```python
from build123d import *

# Parameters (mm, degrees)
SKETCH1_W             = 20
SKETCH1_H             = 20
BOSS_EXTRUDE3_DEPTH   = 30
CUT_EXTRUDE11_REACH   = 39.417
SKETCH10_R            = 0.86
FILLET4_R             = 1
SKETCH12_W            = 2.7
SKETCH12_H            = 30
BOSS_EXTRUDE13_DEPTH  = 25
CUT_EXTRUDE13_REACH   = 51.237
SKETCH14_R            = 3.23
FILLET6_R             = 3
SKETCH16_W            = 2.7
SKETCH16_H            = 30
BOSS_EXTRUDE14_DEPTH  = 25
CUT_EXTRUDE14_REACH   = 51.237
SKETCH17_R            = 3.23
FILLET11_R            = 3
FILLET6_OF_MIRROR1_R  = 3
FILLET11_OF_MIRROR1_R = 3
FILLET12_R            = 1
CUT_EXTRUDE15_REACH   = 57
SKETCH18_R            = 1
CUT_EXTRUDE16_REACH   = 51.237
SKETCH20_R            = 1.98
SKETCH20_R_2          = 1.475
CUT_EXTRUDE17_REACH   = 56.668
SKETCH21_R            = 1.98
SKETCH21_R_2          = 1.475
SKETCH22_R            = 2.725
SKETCH22_R_2          = 3.23
CUT_EXTRUDE18_DEPTH   = 1.35
SKETCH23_R            = 2.725
SKETCH23_R_2          = 3.23
CUT_EXTRUDE19_DEPTH   = 1.35
CUT_EXTRUDE20_REACH   = 52.249
SKETCH24_W            = 8
SKETCH24_H            = 20
FILLET13_R            = 2


with BuildPart() as part:
    # Sketch1 → Boss-Extrude3 (new body)
    with BuildSketch(Plane(origin=(0, 0, 0), x_dir=(1, 0, 0), z_dir=(0, 1, 0))):
        Rectangle(SKETCH1_W, SKETCH1_H)
    extrude(amount=BOSS_EXTRUDE3_DEPTH)

    # Sketch10 → Cut-Extrude11 (cut, up to next)
    with BuildSketch(Plane(origin=(0, 0, -10), x_dir=(-1, 0, 0), z_dir=(0, 0, -1)), mode=Mode.PRIVATE) as cut_extrude11_sk1:
        with Locations((-5.88, 19.86)):
            Circle(SKETCH10_R)
    cut_extrude11_tool1 = extrude(cut_extrude11_sk1.sketch, amount=-CUT_EXTRUDE11_REACH, mode=Mode.PRIVATE) & part.part
    # Sketch10 → Cut-Extrude11 (cut, up to next)
    with BuildSketch(Plane(origin=(0, 0, -10), x_dir=(-1, 0, 0), z_dir=(0, 0, -1)), mode=Mode.PRIVATE) as cut_extrude11_sk2:
        with Locations((-5.92, 9.33)):
            Circle(SKETCH10_R)
    cut_extrude11_tool2 = extrude(cut_extrude11_sk2.sketch, amount=-CUT_EXTRUDE11_REACH, mode=Mode.PRIVATE) & part.part
    # Sketch10 → Cut-Extrude11 (cut, up to next)
    with BuildSketch(Plane(origin=(0, 0, -10), x_dir=(-1, 0, 0), z_dir=(0, 0, -1)), mode=Mode.PRIVATE) as cut_extrude11_sk3:
        Polygon((-1.75, 27.5), (1.75, 27.5), (1.75, 18), (7.3, 18), (7.3, 12), (1.75, 12), (1.75, 2.5), (-1.75, 2.5), (-1.75, 12), (-7.3, 12), (-7.3, 18), (-1.75, 18), align=None)
    cut_extrude11_tool3 = extrude(cut_extrude11_sk3.sketch, amount=-CUT_EXTRUDE11_REACH, mode=Mode.PRIVATE) & part.part
    add(cut_extrude11_tool1.solids().sort_by_distance((5.88, 19.86, -10))[0], mode=Mode.SUBTRACT)
    add(cut_extrude11_tool2.solids().sort_by_distance((5.92, 9.33, -10))[0], mode=Mode.SUBTRACT)
    add(cut_extrude11_tool3.solids().sort_by_distance((0, 15, -10))[0], mode=Mode.SUBTRACT)

    # Fillet4
    fillet4_edges = [part.edges().sort_by_distance(p)[0] for p in [
        (-1.75, 2.5, 0),
        (1.75, 2.5, 0),
        (1.75, 12, 0),
        (7.3, 12, 0),
        (7.3, 18, 0),
        (1.75, 18, 0),
        (1.75, 27.5, 0),
        (-1.75, 27.5, 0),
        (-1.75, 18, 0),
        (-7.3, 18, 0),
        (-7.3, 12, 0),
        (-1.75, 12, 0),
    ]]
    fillet(fillet4_edges, radius=FILLET4_R)

    # Sketch12 → Boss-Extrude13 (add)
    with BuildSketch(Plane.XY.offset(10)):
        with Locations((-8.65, 15)):
            Rectangle(SKETCH12_W, SKETCH12_H)
    boss_extrude13 = extrude(amount=BOSS_EXTRUDE13_DEPTH)

    # Sketch14 → Cut-Extrude13 (cut, up to next)
    with BuildSketch(Plane(origin=(-7.3, 0, 0), x_dir=(0, 0, -1), z_dir=(1, 0, 0)), mode=Mode.PRIVATE) as cut_extrude13_sk1:
        with Locations(Location((-29, 15, 0), (0, 0, 90))):
            Circle(SKETCH14_R)
    cut_extrude13_tool1 = extrude(cut_extrude13_sk1.sketch, amount=-CUT_EXTRUDE13_REACH, mode=Mode.PRIVATE) & part.part
    cut_extrude13 = cut_extrude13_tool1.solids().sort_by_distance((-7.3, 15, 29))[0]
    add(cut_extrude13, mode=Mode.SUBTRACT)

    # Fillet6
    fillet6_edges = [part.edges().sort_by_distance(p)[0] for p in [
        (-8.65, 0, 35),
        (-8.65, 30, 35),
    ]]
    fillet(fillet6_edges, radius=FILLET6_R)

    # Sketch16 → Boss-Extrude14 (add)
    with BuildSketch(Plane(origin=(0, 0, -10), x_dir=(-1, 0, 0), z_dir=(0, 0, -1))):
        with Locations((8.65, 15)):
            Rectangle(SKETCH16_W, SKETCH16_H)
    boss_extrude14 = extrude(amount=BOSS_EXTRUDE14_DEPTH)

    # Sketch17 → Cut-Extrude14 (cut, up to next)
    with BuildSketch(Plane(origin=(-7.3, 0, 0), x_dir=(0, 0, -1), z_dir=(1, 0, 0)), mode=Mode.PRIVATE) as cut_extrude14_sk1:
        with Locations((29, 15)):
            Circle(SKETCH17_R)
    cut_extrude14_tool1 = extrude(cut_extrude14_sk1.sketch, amount=-CUT_EXTRUDE14_REACH, mode=Mode.PRIVATE) & part.part
    cut_extrude14 = cut_extrude14_tool1.solids().sort_by_distance((-7.3, 15, -29))[0]
    add(cut_extrude14, mode=Mode.SUBTRACT)

    # Fillet11
    fillet11_edges = [part.edges().sort_by_distance(p)[0] for p in [
        (-8.65, 30, -35),
        (-8.65, 0, -35),
    ]]
    fillet(fillet11_edges, radius=FILLET11_R)

    # Mirror1: Boss-Extrude13, Cut-Extrude13, Boss-Extrude14, Cut-Extrude14 across plane
    add(boss_extrude13.mirror(Plane(origin=(0, 0, 0), x_dir=(0, 0, 1), z_dir=(1, 0, 0))))
    add(cut_extrude13.mirror(Plane(origin=(0, 0, 0), x_dir=(0, 0, 1), z_dir=(1, 0, 0))), mode=Mode.SUBTRACT)
    add(boss_extrude14.mirror(Plane(origin=(0, 0, 0), x_dir=(0, 0, 1), z_dir=(1, 0, 0))))
    add(cut_extrude14.mirror(Plane(origin=(0, 0, 0), x_dir=(0, 0, 1), z_dir=(1, 0, 0))), mode=Mode.SUBTRACT)

    # Fillet6 of Mirror1
    fillet6_of_mirror1_edges = [part.edges().sort_by_distance(p)[0] for p in [
        (8.65, 0, 35),
        (8.65, 30, 35),
    ]]
    fillet(fillet6_of_mirror1_edges, radius=FILLET6_OF_MIRROR1_R)

    # Fillet11 of Mirror1
    fillet11_of_mirror1_edges = [part.edges().sort_by_distance(p)[0] for p in [
        (8.65, 30, -35),
        (8.65, 0, -35),
    ]]
    fillet(fillet11_of_mirror1_edges, radius=FILLET11_OF_MIRROR1_R)

    # Fillet12
    fillet12_edges = [part.edges().sort_by_distance(p)[0] for p in [
        (0, 0, 10),
        (0, 30, 10),
        (0, 0, -10),
        (0, 30, -10),
    ]]
    fillet(fillet12_edges, radius=FILLET12_R)

    # Sketch18 → Cut-Extrude15 (cut, up to next)
    with BuildSketch(Plane(origin=(0, 0, -10), x_dir=(-1, 0, 0), z_dir=(0, 0, -1)), mode=Mode.PRIVATE) as cut_extrude15_sk1:
        with Locations((-3, 27)):
            Circle(SKETCH18_R)
    cut_extrude15_tool1 = extrude(cut_extrude15_sk1.sketch, amount=-CUT_EXTRUDE15_REACH, mode=Mode.PRIVATE) & part.part
    # Sketch18 → Cut-Extrude15 (cut, up to next)
    with BuildSketch(Plane(origin=(0, 0, -10), x_dir=(-1, 0, 0), z_dir=(0, 0, -1)), mode=Mode.PRIVATE) as cut_extrude15_sk2:
        with Locations((3, 3)):
            Circle(SKETCH18_R)
    cut_extrude15_tool2 = extrude(cut_extrude15_sk2.sketch, amount=-CUT_EXTRUDE15_REACH, mode=Mode.PRIVATE) & part.part
    cut_extrude15_1 = cut_extrude15_tool1.solids().sort_by_distance((3, 27, -10))[0]
    add(cut_extrude15_1, mode=Mode.SUBTRACT)
    cut_extrude15_2 = cut_extrude15_tool2.solids().sort_by_distance((-3, 3, -10))[0]
    add(cut_extrude15_2, mode=Mode.SUBTRACT)
    cut_extrude15 = cut_extrude15_1 + cut_extrude15_2  # Cut-Extrude15 as one shape, for the pattern or mirror that repeats it

    # Mirror2: Cut-Extrude15 across plane
    add(cut_extrude15.mirror(Plane(origin=(0, 0, 0), x_dir=(0, 0, 1), z_dir=(1, 0, 0))), mode=Mode.SUBTRACT)

    # Sketch20 → Cut-Extrude16 (cut, up to next)
    with BuildSketch(Plane.ZY.offset(-7.3), mode=Mode.PRIVATE) as cut_extrude16_sk1:
        with Locations((-13.25, 25.48)):
            Circle(SKETCH20_R)
    cut_extrude16_tool1 = extrude(cut_extrude16_sk1.sketch, amount=-CUT_EXTRUDE16_REACH, mode=Mode.PRIVATE) & part.part
    # Sketch20 → Cut-Extrude16 (cut, up to next)
    with BuildSketch(Plane.ZY.offset(-7.3), mode=Mode.PRIVATE) as cut_extrude16_sk2:
        with Locations((-13.25, 4.52)):
            Circle(SKETCH20_R)
    cut_extrude16_tool2 = extrude(cut_extrude16_sk2.sketch, amount=-CUT_EXTRUDE16_REACH, mode=Mode.PRIVATE) & part.part
    # Sketch20 → Cut-Extrude16 (cut, up to next)
    with BuildSketch(Plane.ZY.offset(-7.3), mode=Mode.PRIVATE) as cut_extrude16_sk3:
        with Locations((-29, 5.48)):
            Circle(SKETCH20_R_2)
    cut_extrude16_tool3 = extrude(cut_extrude16_sk3.sketch, amount=-CUT_EXTRUDE16_REACH, mode=Mode.PRIVATE) & part.part
    # Sketch20 → Cut-Extrude16 (cut, up to next)
    with BuildSketch(Plane.ZY.offset(-7.3), mode=Mode.PRIVATE) as cut_extrude16_sk4:
        with Locations((-29, 24.52)):
            Circle(SKETCH20_R_2)
    cut_extrude16_tool4 = extrude(cut_extrude16_sk4.sketch, amount=-CUT_EXTRUDE16_REACH, mode=Mode.PRIVATE) & part.part
    add(cut_extrude16_tool1.solids().sort_by_distance((7.3, 25.48, -13.25))[0], mode=Mode.SUBTRACT)
    add(cut_extrude16_tool2.solids().sort_by_distance((7.3, 4.52, -13.25))[0], mode=Mode.SUBTRACT)
    add(cut_extrude16_tool3.solids().sort_by_distance((7.3, 5.48, -29))[0], mode=Mode.SUBTRACT)
    add(cut_extrude16_tool4.solids().sort_by_distance((7.3, 24.52, -29))[0], mode=Mode.SUBTRACT)

    # Sketch21 → Cut-Extrude17 (cut, up to next)
    with BuildSketch(Plane(origin=(-7.3, 0, 7.3), x_dir=(0, 0, 1), z_dir=(-1, 0, 0)), mode=Mode.PRIVATE) as cut_extrude17_sk1:
        with Locations(Location((5.95, 25.48, 0), (0, 0, 180))):
            Circle(SKETCH21_R)
    cut_extrude17_tool1 = extrude(cut_extrude17_sk1.sketch, amount=CUT_EXTRUDE17_REACH, mode=Mode.PRIVATE) & part.part
    # Sketch21 → Cut-Extrude17 (cut, up to next)
    with BuildSketch(Plane(origin=(-7.3, 0, 7.3), x_dir=(0, 0, 1), z_dir=(-1, 0, 0)), mode=Mode.PRIVATE) as cut_extrude17_sk2:
        with Locations(Location((5.95, 4.52, 0), (0, 0, 180))):
            Circle(SKETCH21_R)
    cut_extrude17_tool2 = extrude(cut_extrude17_sk2.sketch, amount=CUT_EXTRUDE17_REACH, mode=Mode.PRIVATE) & part.part
    # Sketch21 → Cut-Extrude17 (cut, up to next)
    with BuildSketch(Plane(origin=(-7.3, 0, 7.3), x_dir=(0, 0, 1), z_dir=(-1, 0, 0)), mode=Mode.PRIVATE) as cut_extrude17_sk3:
        with Locations(Location((21.7, 5.48, 0), (0, 0, 180))):
            Circle(SKETCH21_R_2)
    cut_extrude17_tool3 = extrude(cut_extrude17_sk3.sketch, amount=CUT_EXTRUDE17_REACH, mode=Mode.PRIVATE) & part.part
    # Sketch21 → Cut-Extrude17 (cut, up to next)
    with BuildSketch(Plane(origin=(-7.3, 0, 7.3), x_dir=(0, 0, 1), z_dir=(-1, 0, 0)), mode=Mode.PRIVATE) as cut_extrude17_sk4:
        with Locations(Location((21.7, 24.52, 0), (0, 0, 180))):
            Circle(SKETCH21_R_2)
    cut_extrude17_tool4 = extrude(cut_extrude17_sk4.sketch, amount=CUT_EXTRUDE17_REACH, mode=Mode.PRIVATE) & part.part
    add(cut_extrude17_tool1.solids().sort_by_distance((-7.3, 25.48, 13.25))[0], mode=Mode.SUBTRACT)
    add(cut_extrude17_tool2.solids().sort_by_distance((-7.3, 4.52, 13.25))[0], mode=Mode.SUBTRACT)
    add(cut_extrude17_tool3.solids().sort_by_distance((-7.3, 5.48, 29))[0], mode=Mode.SUBTRACT)
    add(cut_extrude17_tool4.solids().sort_by_distance((-7.3, 24.52, 29))[0], mode=Mode.SUBTRACT)

    # Sketch22 → Cut-Extrude18 (cut)
    with BuildSketch(Plane.ZY.offset(-7.3)):
        with Locations(Location((-29, 24.52, 0), (0, 0, 270))):
            Circle(SKETCH22_R)
        with Locations(Location((-13.25, 25.48, 0), (0, 0, 270))):
            Circle(SKETCH22_R_2)
        with Locations(Location((-13.25, 4.52, 0), (0, 0, 270))):
            Circle(SKETCH22_R_2)
        with Locations(Location((-29, 5.48, 0), (0, 0, 270))):
            Circle(SKETCH22_R)
    extrude(amount=-CUT_EXTRUDE18_DEPTH, mode=Mode.SUBTRACT)

    # Sketch23 → Cut-Extrude19 (cut)
    with BuildSketch(Plane(origin=(-7.3, 0, 0), x_dir=(0, 0, -1), z_dir=(1, 0, 0))):
        with Locations((-29, 24.52)):
            Circle(SKETCH23_R)
        with Locations((-13.25, 25.48)):
            Circle(SKETCH23_R_2)
        with Locations((-29, 5.48)):
            Circle(SKETCH23_R)
        with Locations((-13.25, 4.52)):
            Circle(SKETCH23_R_2)
    extrude(amount=-CUT_EXTRUDE19_DEPTH, mode=Mode.SUBTRACT)

    # Sketch24 → Cut-Extrude20 (cut, up to next)
    with BuildSketch(Plane.ZY.offset(10), mode=Mode.PRIVATE) as cut_extrude20_sk1:
        with Locations((-17, 15)):
            Rectangle(SKETCH24_W, SKETCH24_H)
    cut_extrude20_tool1 = extrude(cut_extrude20_sk1.sketch, amount=-CUT_EXTRUDE20_REACH, mode=Mode.PRIVATE) & part.part
    add(cut_extrude20_tool1.solids().sort_by_distance((-10, 15, -17))[0], mode=Mode.SUBTRACT)

    # Fillet13
    fillet13_edges = [part.edges().sort_by_distance(p)[0] for p in [
        (-8.65, 25, -13),
        (-8.65, 5, -13),
        (-8.65, 5, -21),
        (-8.65, 25, -21),
    ]]
    fillet(fillet13_edges, radius=FILLET13_R)


solid = part.part
```
Build history of the part. All positions in model axes, mm. A direction names the side the tool comes from. Round coordinates to 2 decimals unless told otherwise and drop trailing zeros. Order: outer loops, then holes, each group sorted by start corner. A loop starts at its lowest first (then second) coordinate and runs counter-clockwise, first axis right, second up. Notation, with made-up numbers: (36, -26.75) -> (66, -26.75) arc R34 cw to (66, 6.25) -> close; hole circle Ø7 at (73, 4.5). An arc over 180 degrees is marked (long way). Answer in a Markdown table with one row per item.
1) Pin check, flat tips, straight feed: P1, Ø9.5, axis at x = 1.5, y = 25, coming from the -Z side; P2, Ø2, axis at x = 5.92, y = 9.33, coming from the +Z side; P3, Ø6, axis at x = -6, y = 22, coming from the -Z side. Stop position of each tip, or through.
Values:
| item | result |
|---|---|
| P1 | z = -10 |
| P2 | z = 10 |
| P3 | z = -35 |
2) Wall check: L1, parallel to Y at x = 9.1, z = -29 (3 decimals); L2, parallel to Y at x = -3, z = 2.25; L3, parallel to Y at x = -7.6, z = 13.25. Give the ranges that are in metal, low to high.
Values:
| item | result |
|---|---|
| L1 | 0 to 4.005, 6.955 to 11.77, 18.23 to 23.045, 25.995 to 30 |
| L2 | 0 to 2, 4 to 12, 18 to 26, 28 to 30 |
| L3 | 0 to 1.29, 7.75 to 22.25, 28.71 to 30 |
3) Band-saw the part on D-D on z = -4.5. Give the number of separate pieces and of enclosed holes in the cut face, and give its area (3 significant figures).
Values:
| item | result |
|---|---|
| separate pieces | 1 |
| enclosed holes | 7 |
| area | 430 mm2 |
4) Band-saw the part on B-B on y = 9.33. Give the cut face in (x, z).
Values:
| item | result |
|---|---|
| outline | (-10, -35) -> (-7.3, -35) -> (-7.3, -21) -> (-10, -21) -> close; (-10, -13) -> (-7.3, -13) -> (-7.3, -10) -> (-1.75, -10) -> (-1.75, 10) -> (-7.3, 10) -> (-7.3, 35) -> (-10, 35) -> close; (1.75, -10) -> (5.06, -10) -> (5.06, 10) -> (1.75, 10) -> close; (6.78, -10) -> (7.3, -10) -> (7.3, -35) -> (10, -35) -> (10, 35) -> (7.3, 35) -> (7.3, 10) -> (6.78, 10) -> close |
5) Mould opens along Y. For faces 4 (the flat face through (9, 15, 35)), 5 (the cylindrical face through (8.63, 0.86, 34.1)), 6 (the cylindrical face through (2.263, 3.676, -0.14)) say: released by +Y, released by -Y, zero draft, split by the parting line, or undercut.
Values:
| item | result |
|---|---|
| face 4 | zero draft |
| face 5 | released by -Y |
| face 6 | undercut |
6) Band-saw the part on A-A on z = 20. Give the cut face in (x, y).
Values:
| item | result |
|---|---|
| outline | (-10, 0) -> (-7.3, 0) -> (-7.3, 30) -> (-10, 30) -> close; (7.3, 0) -> (10, 0) -> (10, 30) -> (7.3, 30) -> close |
7) Band-saw the part on C-C on x = -5. Give the cut face in (y, z).
Values:
| item | result |
|---|---|
| outline | (0, -9) arc R1 ccw to (1, -10) -> (12, -10) -> (12, 10) -> (1, 10) arc R1 ccw to (0, 9) -> close; (18, -10) -> (29, -10) arc R1 ccw to (30, -9) -> (30, 9) arc R1 ccw to (29, 10) -> (18, 10) -> close |
8) Which spindle directions (+Z, -Z, +X, -X, +Y, -Y) get a long thin tool onto all of the face, cutting with end or side? Do faces 1 (the flat face through (8.65, 23, -30)), 2 (the cylindrical face through (-9.32, 25.42, 30.17)), 3 (the flat face through (-5, 18, 0)). Say none if no direction does.
Values:
| item | result |
|---|---|
| face 1 | none |
| face 2 | -X |
| face 3 | +Z, -Z |
